Autodesk Fusion 360 part; units mm, degrees
sketch "Sketch1" plane through (0, 0, 0) normal (0, 1, 0) x (1, 0, 0)
  circle A0 centre (0, 0) radius 15
  circle A1 centre (0, 0) radius 17.5
  dimension "d1" = 30
  dimension "d2" = 35
extrude "Extrude1" add sketch "Sketch1" along normal blind 20
sketch "Sketch2" plane through (0, 20, 0) normal (0, 1, 0) x (-1, 0, 0)
  circle A0 centre (0, 0) radius 15
  circle A1 centre (0, 0) radius 17.5
  circle A2 centre (0, 0) radius 16.5
  circle A3 centre (0, 0) radius 17.5
  circle A4 centre (0, 0) radius 19
  circle A5 centre (0, 0) radius 20
  dimension "d5" = 33
  dimension "d10" = 38
  dimension "d13" = 40
extrude "Extrude2" cut sketch "Sketch2" against normal blind 20 contours A1 A3
extrude "Extrude3" add sketch "Sketch2" against normal blind 2 contours A1 A3
extrude "Extrude4" add sketch "Sketch2" against normal blind 4 contours A1 A3 | A4
extrude "Extrude5" add sketch "Sketch2" against normal blind 4 contours A5
sketch "Sketch3" plane through (0, 0, 0) normal (0, -1, 0) x (1, 0, 0)
  circle A0 centre (0, 0) radius 16.5
  circle A1 centre (0, 0) radius 15
  circle A2 centre (0, 0) radius 16
  circle A3 centre (0, 0) radius 16.5
extrude "Extrude6" cut sketch "Sketch3" against normal blind 16 contours A0 A3
fillet "Fillet1" radius 4 1 edges at (18.6465, 20, -7.2323)
For this review, take the finished solid that the model builds, in its own axes (mm). Give positions to 0.01 mm unless a question says otherwise; leave off trailing zeros. Loops run counter-clockwise (first coordinate to the right, second up) from the corner with the lowest first, then second, coordinate; pieces in that order, holes last. Notation, with made-up numbers: M -15,58 L 24,58 A18 cw 24,69 Z; hole C -20,-33.5 d5. An arc over 180 degrees is marked long. One line per item, written item: value. Start each with the question number.
Q1. Draft analysis for pull direction X (two halves, no side actions). For faces 1 (the face through (8.98, 16, 13.43)), 2 (the face through (-3.47, 7.89, -15.62)), 3 (the face through (-14.985, 9.86, 0.66)), state which applies: released by +X, released by -X, zero draft, split by the parting line, or undercut.
Q2. Add section D-D (y = 17.25). Give the boundary of the cut face in (x, z).
Q3. Add section C-C (y = 1.25). Give the boundary of the cut face in (x, z).
Q4. For L1, parallel to Z at x = 0, y = 12; L2, parallel to Z at x = -3.5, y = 10; L3, parallel to X at y = 3.5, z = -11.5, list the stretches that pass through material, from the lowest coordinate up.
Q5. Clearance check with flat-ended pins moving along their axes: pin 1 Ø12 at (y, z) = (4.5, 5.5) entering from -X; pin 2 Ø1 at (x, y) = (-14, 16) entering from -Z; pin 3 Ø6 at (x, y) = (5.5, 9) entering from +Z. State where each tip first meets the part, or that it passes through.
Reply:
1. face 1: zero draft
1. face 2: split by the parting line
1. face 3: undercut
2. outline: C 0,0 d39.6; hole C 0,0 d30
3. outline: C 0,0 d32; hole C 0,0 d30
4. L1: -16 to -15, 15 to 16
4. L2: -15.61 to -14.59, 14.59 to 15.61
4. L3: -11.12 to -9.63, 9.63 to 11.12
5. pin 1: x = -16
5. pin 2: z = -14.76
5. pin 3: z = 15.8
